from build123d import *

# Parameters (mm, degrees)
PROFILEBOSS_EXTRUDE1_DEPTH           = 80
SKETCH2_R                            = 2.3
LEDSTRIPMOUNTHOLESCUT_EXTRUDE1_DEPTH = 4.5
SKETCH4_W                            = 28
SKETCH4_H                            = 11.5
POWERCONNECTORCUT_EXTRUDE4_DEPTH     = 6.5
SKETCH3_R                            = 2.3
MOUNTINGHOLESCUT_EXTRUDE3_DEPTH      = 4.5


with BuildPart() as part:
    # Sketch1 → ProfileBoss-Extrude1 (new body)
    with BuildSketch(Plane(origin=(0, 0, 0), x_dir=(0, 0, -1), z_dir=(1, 0, 0))):
        with BuildLine():
            Line((0, 0), (5.499461553, 0))
            ThreePointArc((5.499461553, 0), (6.914055855, 0.585944145), (7.5, 2.000538447))
            Line((7.5, 2.000538447), (7.5, 3.5))
            Line((7.5, 3.5), (17.922539551, 8.36011001))
            Line((17.922539551, 8.36011001), (19.190394336, 5.641186649))
            ThreePointArc((19.190394336, 5.641186649), (20.700753359, 6.16912635), (21.340729536, 7.635528477))
            Line((21.340729536, 7.635528477), (21.340729536, 13.36011001))
            ThreePointArc((21.340729536, 13.36011001), (20.754943098, 14.774323572), (19.340729536, 15.36011001))
            Line((19.340729536, 15.36011001), (0, 15.36011001))
            Line((0, 15.36011001), (0, 0))
        make_face()
    extrude(amount=PROFILEBOSS_EXTRUDE1_DEPTH)

    # Sketch2 → LedStripMountHolesCut-Extrude1 (cut)
    with BuildSketch(Plane(origin=(0, 0.002211655, 0.001031312), x_dir=(1, 0, 0), z_dir=(0, -0.906307787036651, -0.4226182617406973))):
        with Locations(Location((36.15, -14.026472319, 0), (0, 0, 270))):
            Circle(SKETCH2_R)
    extrude(amount=-LEDSTRIPMOUNTHOLESCUT_EXTRUDE1_DEPTH, mode=Mode.SUBTRACT)

    # Sketch4 → PowerConnectorCut-Extrude4 (cut)
    with BuildSketch(Plane(origin=(0, 0.002211655, 0.001031312), x_dir=(1, 0, 0), z_dir=(0, -0.906307787036651, -0.4226182617406973))):
        with Locations((14, -14.026472319)):
            Rectangle(SKETCH4_W, SKETCH4_H)
    extrude(amount=-POWERCONNECTORCUT_EXTRUDE4_DEPTH, mode=Mode.SUBTRACT)

    # Sketch3 → MountingHolesCut-Extrude3 (cut)
    with BuildSketch(Plane.XY):
        with Locations((50, 10.86011001)):
            Circle(SKETCH3_R)
    extrude(amount=-MOUNTINGHOLESCUT_EXTRUDE3_DEPTH, mode=Mode.SUBTRACT)


solid = part.part
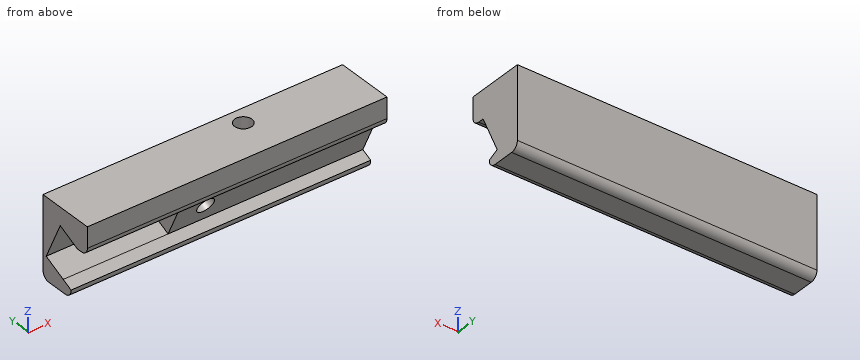
Could you check a few things on this model? Use its own coordinates, in mm. Give positions to 0.01 mm unless a question says otherwise; leave off trailing zeros. Order: outer loops, then holes, each group sorted by start corner. A loop starts at its lowest first (then second) coordinate and runs counter-clockwise, first axis right, second up.
Item 1: If we section it at B-B, the plane x = 9.5: Write out the boundary of the cut face in (y, z), plus the area to 3 significant figures.
Item 2: If we section it at C-C, the plane x = 50: Write out the boundary of the cut face in (y, z).
Item 3: I need wall thicknesses on line 1 (Y direction, x = 50, z = -3.3); line 2 (Z direction, x = 25, y = 3); line 3 (Z direction, x = 25, y = 11.5). Which ranges of each line are inside material? Lowest first, please.
Item 4: If we section it at A-A, the plane x = 73: Write out the boundary of the cut face in (y, z).
Item 5: I'm going to push flat-ended pins straight in: pin 1 (1.4 mm diameter, centred on x = 49.5, y = 10, fed in from +Z); pin 2 (1.5 mm diameter, centred on x = 47, y = 2.5, fed in from -Z); pin 3 (12 mm diameter, centred on x = 9.5, z = -14, fed in from -Y). Where does each tip first touch, or does it pass through?
Values:
1. outline: (0, -5.5) arc R2 ccw to (2, -7.5) - (3.5, -7.5) - (9.39, -4.75) - (14.25, -15.18) - (5.64, -19.19) arc R2 ccw to (7.64, -21.34) - (13.36, -21.34) arc R2 ccw to (15.36, -19.34) - (15.36, 0) - (0, 0) - close
1. area: 168 mm2
2. outline: (0, -5.5) arc R2 ccw to (2, -7.5) - (3.5, -7.5) - (8.36, -17.92) - (5.64, -19.19) arc R2 ccw to (7.64, -21.34) - (13.36, -21.34) arc R2 ccw to (15.36, -19.34) - (15.36, 0) - (13.16, 0) - (13.16, -4.5) - (8.56, -4.5) - (8.56, 0) - (0, 0) - close
3. line 1: y = 0 to 8.56, 13.16 to 15.36
3. line 2: z = -7.5 to 0
3. line 3: z = -21.34 to -16.46, -9.28 to 0
4. outline: (0, -5.5) arc R2 ccw to (2, -7.5) - (3.5, -7.5) - (8.36, -17.92) - (5.64, -19.19) arc R2 ccw to (7.64, -21.34) - (13.36, -21.34) arc R2 ccw to (15.36, -19.34) - (15.36, 0) - (0, 0) - close
5. pin 1: stops at z = -4.5
5. pin 2: stops at z = -7.5
5. pin 3: stops at y = 5.64
